Verification items for this drawing (mm, ordinates from the low corner). A direction names the side the tool comes from. Round coordinates to 2 decimals unless told otherwise and drop trailing zeros. Loops run counter-clockwise (first coordinate to the right, second up) from the corner with the lowest first, then second, coordinate; pieces in that order, holes last. Notation, with made-up numbers: M 11,33 L 55,33 A16 ccw 55,62 Z; hole C 46,71.5 d11. An arc over 180 degrees is marked long. Write item = value, one per line.
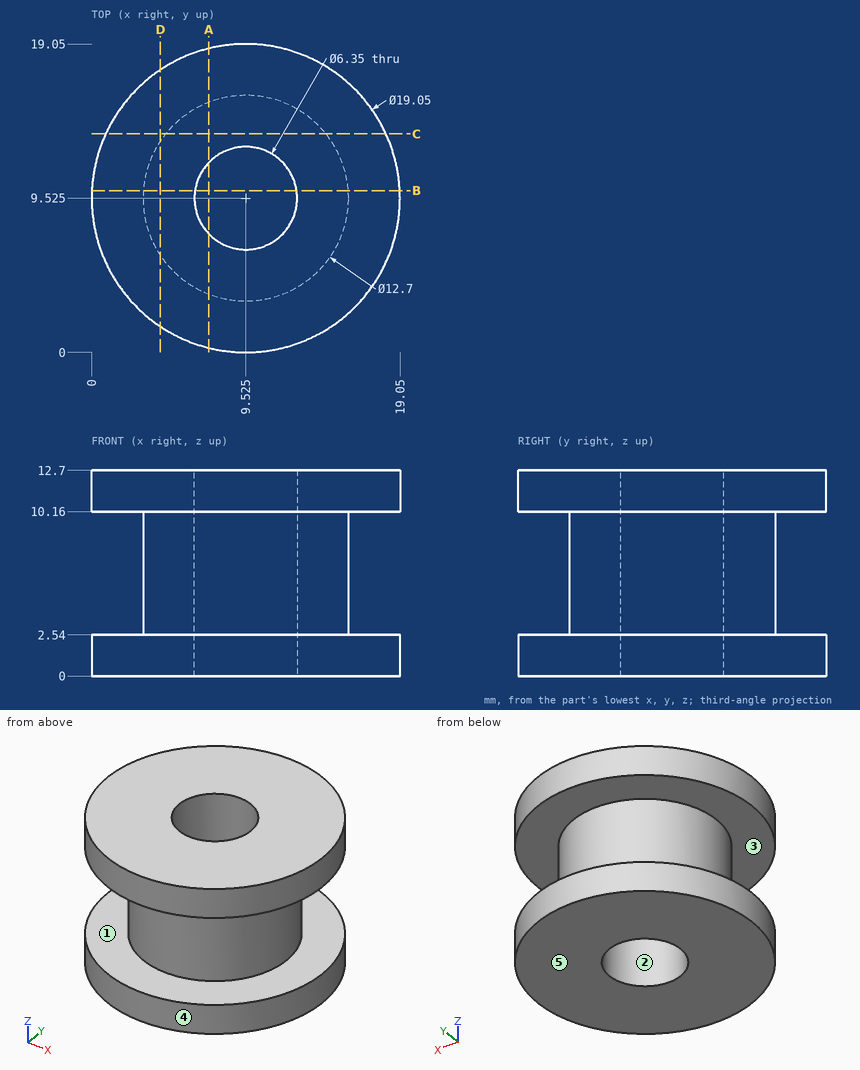
(1) Sectioned sample at B-B on y = 10. Record the cut outline in (x, z).
Result set:
outline = M 0.01,0 L 6.39,0 L 6.39,12.7 L 0.01,12.7 L 0.01,10.16 L 3.19,10.16 L 3.19,2.54 L 0.01,2.54 Z; M 12.66,0 L 19.04,0 L 19.04,2.54 L 15.86,2.54 L 15.86,10.16 L 19.04,10.16 L 19.04,12.7 L 12.66,12.7 Z
(2) Sectioned sample at A-A on x = 7.25. Record the cut outline in (y, z).
Result set:
outline = M 0.28,0 L 7.31,0 L 7.31,12.7 L 0.28,12.7 L 0.28,10.16 L 3.6,10.16 L 3.6,2.54 L 0.28,2.54 Z; M 11.74,0 L 18.77,0 L 18.77,2.54 L 15.45,2.54 L 15.45,10.16 L 18.77,10.16 L 18.77,12.7 L 11.74,12.7 Z
(3) Material ranges on line 1 along Z through (x, y) = (16.25, 11.25); line 2 along X through (y, z) = (12.25, 7.5); line 3 along X through (y, z) = (7.5, 2.25), recorded low to high. Write a range as from..to.
Result set:
line_1 = 0..2.54, 10.16..12.7
line_2 = 3.79..7.9, 11.15..15.26
line_3 = 0.22..7.08, 11.97..18.83
(4) Tool access check on the marked faces 1 and 2. Record the directions out of +Z, -Z, +X, -X, +Y, -Y that give a thin tool (end or side, any length) a straight path to the whole face; none if there is none.
Result set:
face_1 = none
face_2 = +Z, -Z
(5) Sectioned sample at D-D on x = 4.25. Record the cut outline in (y, z).
Result set:
outline = M 1.59,0 L 17.46,0 L 17.46,2.54 L 13.06,2.54 L 13.06,10.16 L 17.46,10.16 L 17.46,12.7 L 1.59,12.7 L 1.59,10.16 L 5.99,10.16 L 5.99,2.54 L 1.59,2.54 Z
(6) Sectioned sample at C-C on y = 13.5. Record the cut outline in (x, z).
Result set:
outline = M 0.87,0 L 18.18,0 L 18.18,2.54 L 14.48,2.54 L 14.48,10.16 L 18.18,10.16 L 18.18,12.7 L 0.87,12.7 L 0.87,10.16 L 4.57,10.16 L 4.57,2.54 L 0.87,2.54 Z
(7) Release check for a two-part mould opening along Z. For the marked faces 3, 4 and 5 record: released by +Z, released by -Z, zero draft, split by the parting line, or undercut.
Result set:
face_3 = undercut
face_4 = zero draft
face_5 = released by -Z
(8) Depth check by flat-ended pin: pin 1 Ø3 at (y, z) = (11, 6) entering from +X (3 decimals); pin 2 Ø1 at (x, z) = (9, 3) entering from +Y; pin 3 Ø6 at (y, z) = (2.5, 3.5) entering from -X; pin 4 Ø5.5 at (x, y) = (9.525, 9.525) entering from +Z (3 decimals). Enter the tip coordinate at first touch or a pass-through.
Result set:
pin_1 = 15.875
pin_2 = 19.04
pin_3 = 0.97
pin_4 = through
